from build123d import *

# Parameters (mm, degrees)
F4_ANGLE_BACK   = 15
F4_ANGLE        = 30
F4_COPIES_COUNT = 5


# Not quite as in the source:
# - a pattern or mirror of a feature is missing from the dataset's text; its kind, count and spacing are read off the source's solid


with BuildPart() as f2:
    # F1 (on Front) → F2 (revolve)
    with BuildSketch(Plane.XZ):
        with BuildLine():
            Line((40, 6), (40, 0))
            Line((40, 0), (50, 0))
            Line((50, 0), (50, 12.9))
            Line((50, 12.9), (46.9, 12.9))
            ThreePointArc((46.9, 12.9), (44.8790367902, 8.0209632098), (40, 6))
        make_face()
    revolve(axis=Axis((0, 0, 7.8032705933), (0, 0, 1)))

    # F3 (on Front) → F4 (revolve)
    with BuildSketch(Plane.XZ, mode=Mode.PRIVATE) as f4_sk:
        Polygon((50, 35), (50, 0), (76, 0), (54, 35), align=None)
        Polygon((53, 30.9536291067), (70.5708525814, 3), (53, 3), align=None, mode=Mode.SUBTRACT)
    f4 = revolve(f4_sk.sketch.rotate(Axis((0, 0, 7.8032705933), (0, 0, 1)), -F4_ANGLE_BACK), axis=Axis((0, 0, 7.8032705933), (0, 0, 1)), revolution_arc=F4_ANGLE)

    # F4_copies: F4 ×5 about axis
    f4_copies_axis = Axis((0, 0, 0), (0, 0, 1))
    for i in range(1, F4_COPIES_COUNT):
        add(f4.rotate(f4_copies_axis, i * 360 / F4_COPIES_COUNT))


solid = f2.part
Work out the finished part from the listing and answer in its coordinate system (mm). A direction names the side the tool comes from. Give positions to 0.01 mm unless a question says otherwise; leave off trailing zeros. Order: outer loops, then holes, each group sorted by start corner. A loop starts at its lowest first (then second) coordinate and runs counter-clockwise, first axis right, second up. Notation, with made-up numbers: M 18.5,-29.5 L 77.5,-29.5 A21 cw 77.5,3.5 Z; hole C 86.25,76.5 d2. An arc over 180 degrees is marked long. Return JSON: item names as keys, results as strings.
Q1. Each of these flat-tipped pins is pushed along its axis until it touches: pin 1 (2 mm diameter, centred on y = -34, z = 8, fed in from -X); pin 2 (16.5 mm diameter, centred on x = -54, y = 33.5, fed in from +Z); pin 3 (21 mm diameter, centred on x = 18, y = 63.5, fed in from +Z). Where does it stop, or does it pass through?
Answer below:
{"pin 1": "stops at x = -63.19", "pin 2": "stops at z = 32.94", "pin 3": "stops at z = 32.61"}
Q2. The mould has two halves that part along Y. Classify faces 6 (the face through (-52.321, 38.308, 17.745)), 7 (the face through (-42.763, 31.31, 17.172)), 8 (the face through (16, 49, 35)), 9 (the face through (33.755, 51.978, 17.582)): pulls with the +Y half, pulls with the -Y half, needs draft (parallel to the pull), parting line crosses it, or undercut.
Answer below:
{"face 6": "pulls with the +Y half", "face 7": "undercut", "face 8": "needs draft", "face 9": "undercut"}
Q3. Find the intervals of material crossed by line 1 along Y through (x, z) = (20, 23.5); line 2 along X through (y, z) = (-41.5, 11); line 3 along Y through (x, z) = (15.5, 23.5), in increasing order. Write a range as [from, to].
Answer below:
{"line 1": "y = [-57.87, -54.11], [-49.08, -45.83], [45.83, 49.08], [54.11, 57.87]", "line 2": "x = [-55.23, -50.73], [-27.89, -21.27], [21.27, 27.89]", "line 3": "y = [-59.23, -55.56], [-50.68, -47.54], [47.54, 50.68], [55.56, 59.23]"}
Q4. Find section A-A, the plane y = 0. Write down the section's boundary in (x, z), and give its area (3 significant figures).
Answer below:
{"outline": "M -50,0 L -40,0 L -40,6 A6.9 cw -46.9,12.9 L -50,12.9 Z; M 40,0 L 76,0 L 54,35 L 50,35 L 50,12.9 L 46.9,12.9 A6.9 cw 40,6 Z; hole M 53,3 L 70.57,3 L 53,30.95 Z", "area": "463 mm^2"}
Q5. Find section C-C, the plane z = 23.5. State how many separate pieces and enclosed holes the cut face has, and give its area (3 significant figures).
Answer below:
{"separate pieces": "10", "enclosed holes": "0", "area": "956 mm^2"}
Q6. Which of the six approach directions +Z, -Z, +X, -X, +Y, -Y give full straight-line access (tool end or side, diameter ignored) to faces 1 (the face through (-40, 30, 24)), 2 (the face through (-57.86, -22.21, 17.58)), 3 (the face through (16.193, -50.466, 17.172)), 4 (the face through (15.3, -47.6, 23.8)), 5 (the face through (33.755, -51.978, 17.582))?
Answer below:
{"face 1": "+Z, +X", "face 2": "+Z, -Z, -X", "face 3": "none", "face 4": "+Z", "face 5": "+Z, -Z, +X"}
Q7. Find section B-B, the plane x = 0. Write down the section's boundary in (y, z).
Answer below:
{"outline": "M -50,0 L -40,0 L -40,6 A6.9 cw -46.9,12.9 L -50,12.9 Z; M 40,0 L 50,0 L 50,12.9 L 46.9,12.9 A6.9 cw 40,6 Z"}
